The listing builds one solid part. Answer for the finished solid, in the listing's coordinates (mm). A direction names the side the tool comes from. Coordinates: 2 decimals unless noted, no trailing zeros. Write each loop counter-clockwise with the first axis right and the second up, starting at its lowest first coordinate (ties: lowest second). Pieces come first, ordered by that corner, then holes.
```python
from build123d import *

# Parameters (mm, degrees)
MAIN_DEPTH            = 4.7625
MAIN_DEPTH_BACK       = 4.7625
SKETCH1_W             = 38.1
SKETCH1_H             = 31.75
FILLET_2_R            = 4.7625
SERVOHORNPOCKET_DEPTH = 3.81


with BuildPart() as part:
    # Sketch1 → Main (new, two sides: drawn at the far end of the back side and taken through both)
    with BuildSketch(Plane.XY.offset(-MAIN_DEPTH_BACK)):
        with Locations((0, -7.9375)):
            Rectangle(SKETCH1_W, SKETCH1_H)
    extrude(amount=MAIN_DEPTH + MAIN_DEPTH_BACK)

    # Fillet 2
    fillet_2_edges = [part.edges().sort_by_distance(p)[0] for p in [
        (0, 7.9375, -4.7625),
        (0, 7.9375, 4.7625),
    ]]
    fillet(fillet_2_edges, radius=FILLET_2_R - 0.0001)  # a hair under: the kernel refuses the full size

    # Sketch2 → ServoHornPocket (cut)
    with BuildSketch(Plane.ZY.offset(19.05)):
        with BuildLine():
            Line((3.681584666, 2.768121212), (2.240359567, -10.272598485))
            ThreePointArc((2.240359567, -10.272598485), (0, -12.279), (-2.240359567, -10.272598485))
            Line((-2.240359567, -10.272598485), (-3.530690742, 4.294749474))
            ThreePointArc((-3.530690742, 4.294749474), (0.767033706, 6.798710156), (3.681584666, 2.768121212))
        make_face()
    extrude(amount=-SERVOHORNPOCKET_DEPTH, mode=Mode.SUBTRACT)


solid = part.part
```
(1) Section A-A, the plane y = 2 is taken. Write down the section's boundary in (x, z), plus the area to 3 significant figures.
(2) This flat-tipped pin is pushed along its axis until it touches: pin 1 (4 mm diameter, centred on y = -6, z = -0.5, fed in from -X). Where does it stop, or does it pass through?
(3) Section B-B, the plane z = 3 is taken. Write down the section's boundary in (x, y).
(4) Find the intervals of material crossed by probe 1 along X at (y, z) = (-10, 1); probe 2 along Z at (x, y) = (-17, 1); probe 3 along Y at (x, z) = (-0.5, 2), in increasing order.
(5) For a pull along Z with two mould halves and no side action, classify faces 1 (the flat face through (19.05, -8, 0)), 2 (the flat face through (0, -10, -4.762)), 3 (the cylindrical face through (-17.172, 6.814, 0.692)) as pulls with the +Z half, pulls with the -Z half, needs draft (parallel to the pull), parting line crosses it, or undercut.
(6) Which of the six approach directions +Z, -Z, +X, -X, +Y, -Y give full straight-line access (tool end or side, diameter ignored) to faces 4 (the flat face through (-15.24, -3, 0)), 5 (the cylindrical face through (0.27, 6.58, -3.33))?
Solution:
1. outline: (-19.05, -4.76) - (19.05, -4.76) - (19.05, 4.76) - (-19.05, 4.76) - (-19.05, 3.6) - (-15.24, 3.6) - (-15.24, -3.33) - (-19.05, -3.33) - close
1. area: 337 mm2
2. pin 1: stops at x = -15.24
3. outline: (-19.05, -23.81) - (19.05, -23.81) - (19.05, 6.87) - (-19.05, 6.87) - (-19.05, 5.35) - (-15.24, 5.35) - (-15.24, -3.4) - (-19.05, -3.4) - close
4. probe 1: x = -15.24 to 19.05
4. probe 2: z = -4.76 to -3.24, 3.49 to 4.76
4. probe 3: y = -23.81 to 7.5
5. face 1: needs draft
5. face 2: pulls with the -Z half
5. face 3: undercut
6. face 4: -X
6. face 5: -Z, +X, -X, +Y
